from build123d import *

# Parameters (mm, degrees)
F1_DEPTH = 20


with BuildPart() as f1:
    # F0 (on Front) → F1 (new body)
    with BuildSketch(Plane.XZ):
        with BuildLine():
            ThreePointArc((-18.656017, 14.463057), (-18.708848, 14.556927), (-18.760553, 14.651424))
            ThreePointArc((-18.760553, 14.651424), (-74.939471, 0), (-18.760553, -14.651424))
            ThreePointArc((-18.760553, -14.651424), (-18.708848, -14.556927), (-18.656017, -14.463057))
            ThreePointArc((-18.656017, -14.463057), (-15.883459, -7.46647), (-14.939471, 0))
            ThreePointArc((-14.939471, 0), (-15.883459, 7.46647), (-18.656017, 14.463057))
        make_face()
        Polygon((-51.569248, 17.787172), (-47.052302, 21.037134), (-30.079958, 13.386369), (-27.777194, 12.348333), (-26.537009, 0), (-25.664363, -8.688802), (-42.82664, -21.037134), (-62.101748, -12.348333), (-64.21458, 8.688802), align=None, mode=Mode.SUBTRACT)
        with BuildLine():
            ThreePointArc((70.44672, 14.651424), (70.040505, 14.235547), (69.618481, 13.835724))
            ThreePointArc((69.618481, 13.835724), (64.060529, 0), (69.618481, -13.835724))
            ThreePointArc((69.618481, -13.835724), (70.040505, -14.235547), (70.44672, -14.651424))
            ThreePointArc((70.44672, -14.651424), (92.051894, -18.334069), (104.060529, 0))
            ThreePointArc((104.060529, 0), (101.772313, 9.289387), (95.431258, 16.453161))
            ThreePointArc((95.431258, 16.453161), (82.621982, 19.948198), (70.44672, 14.651424))
        make_face()
        Polygon((89.50246, 14.579673), (91.770843, 11.156633), (99.608271, -0.670217), (88.227631, -14.99389), (71.088197, -8.596516), (71.458768, 0), (71.876085, 9.680951), align=None, mode=Mode.SUBTRACT)
        with BuildLine():
            ThreePointArc((-12.005609, 10), (-15.854632, 11.450985), (-18.656017, 14.463057))
            ThreePointArc((-18.656017, 14.463057), (-15.883459, 7.46647), (-14.939471, 0))
            ThreePointArc((-14.939471, 0), (-15.883459, -7.46647), (-18.656017, -14.463057))
            ThreePointArc((-18.656017, -14.463057), (-15.854632, -11.450985), (-12.005609, -10))
            Line((-12.005609, -10), (57.99466, -10))
            ThreePointArc((57.99466, -10), (59.515113, -9.922742), (61.035567, -10))
            ThreePointArc((61.035567, -10), (65.635285, -11.228089), (69.618481, -13.835724))
            ThreePointArc((69.618481, -13.835724), (64.060529, 0), (69.618481, 13.835724))
            ThreePointArc((69.618481, 13.835724), (65.635285, 11.228089), (61.035567, 10))
            ThreePointArc((61.035567, 10), (59.515113, 9.922742), (57.99466, 10))
            Line((57.99466, 10), (-12.005609, 10))
        make_face()
        with BuildLine():
            ThreePointArc((-7.005609, -4.890676), (-12.005609, 0.109324), (-7.005609, 5.109324))
            Line((-7.005609, 5.109324), (52.994391, 5.109324))
            ThreePointArc((52.994391, 5.109324), (57.994391, 0.109324), (52.994391, -4.890676))
            Line((52.994391, -4.890676), (-7.005609, -4.890676))
        make_face(mode=Mode.SUBTRACT)
    extrude(amount=F1_DEPTH)


solid = f1.part
CAD build for the part. Positions are in the model's coordinates, mm. A direction names the side the tool comes from. Give positions to 0.01 mm unless a question says otherwise; leave off trailing zeros. Loops run counter-clockwise (first coordinate to the right, second up) from the corner with the lowest first, then second, coordinate; pieces in that order, holes last. Notation, with made-up numbers: M 10.5,-10 L 46.5,-10 A16 cw 46.5,-6 Z; hole C 5.25,16.25 d7. An arc over 180 degrees is marked long. Write each question's results on one line, items separated by ' | '.
Q1. Band-saw the part on A-A on x = -3.5. Write the cut outline in (y, z), and give its area (3 significant figures).
Geometry check:
outline: M -20,-10 L 0,-10 L 0,-4.89 L -20,-4.89 Z; M -20,5.11 L 0,5.11 L 0,10 L -20,10 Z | area: 200 mm²
Q2. Band-saw the part on C-C on y = -5.75. Give the number of separate pieces and of enclosed holes in the cut face, and give its area (3 significant figures).
Geometry check:
separate pieces: 1 | enclosed holes: 3 | area: 3,300 mm²
Q3. Which spindle directions (+Z, -Z, +X, -X, +Y, -Y) get a long thin tool onto all of the face, cutting with end or side? Do faces 4 (the face through (-15.81, -9.86, 11.42)), 5 (the face through (1, 0, 7)), 6 (the face through (-15.9, -9.86, -11.48)), 7 (the face through (-12.004, -9.86, -0.001)). Say none if no direction does.
Geometry check:
face 4: +Z, +Y, -Y | face 5: +Z, -Z, +X, -X, +Y | face 6: -Z, +Y, -Y | face 7: +Y, -Y
Q4. Mould opens along Z. For faces 1 (the face through (79.78, -9.86, -11.84)), 2 (the face through (65.57, -9.86, -11.2)), 3 (the face through (59.536, -9.86, 9.923)) say: pulls with the +Z half, pulls with the -Z half, needs draft (parallel to the pull), parting line crosses it, or undercut.
Geometry check:
face 1: undercut | face 2: pulls with the -Z half | face 3: pulls with the +Z half
Q5. Band-saw the part on D-D on x = -58. Write the cut outline in (y, z), and give its area (3 significant figures).
Geometry check:
outline: M -20,-27.01 L 0,-27.01 L 0,-14.2 L -20,-14.2 Z; M -20,13.16 L 0,13.16 L 0,27.01 L -20,27.01 Z | area: 533 mm²
Q6. Band-saw the part on B-B on z = 2.5. Write the cut outline in (x, y), and give its area (3 significant figures).
Geometry check:
outline: M -74.84,-20 L -63.59,-20 L -63.59,0 L -74.84,0 Z; M -26.79,-20 L -11.4,-20 L -11.4,0 L -26.79,0 Z; M 57.39,-20 L 71.57,-20 L 71.57,0 L 57.39,0 Z; M 97.51,-20 L 103.9,-20 L 103.9,0 L 97.51,0 Z | area: 944 mm²
Q7. Flat gauge pins, fed straight in: P1, Ø8, axis at x = -12, y = -17.5, coming from the +Z side; P2, Ø2, axis at x = 66.5, y = -10.5, coming from the -Z side; P3, Ø12, axis at y = -3, z = 16.5, coming from the +X side. Where does each tip first touch, or does it go through?
Geometry check:
P1: stops at z = 11.55 | P2: stops at z = -12.22 | P3: stops at x = 101.08
Q8. Probe probe 1 along Z at (x, y) = (32, -14); probe 2 along X at (y, z) = (-7.5, 23); probe 3 along X at (y, z) = (-12.5, 6). List the from-to ranges inside material, lowest first.
Geometry check:
probe 1: z = -10 to -4.89, 5.11 to 10 | probe 2: x = -64.2 to -25.68 | probe 3: x = -74.33 to -63.94, -27.14 to 71.72, 95.19 to 103.14
